Part print with two shaded views. Sizes in mm from the minimum x, y, z corner. A direction names the side the tool comes from. Give positions to 0.01 mm unless a question says otherwise; leave off trailing zeros. Loops run counter-clockwise (first coordinate to the right, second up) from the corner with the lowest first, then second, coordinate; pieces in that order, holes last. Notation, with made-up numbers: (63.5, -27) -> (111.5, -27) arc R20 ccw to (111.5, -10) -> close; hole circle Ø7 at (-33, -40). An arc over 180 degrees is marked (long way). One line per question, with ' | ' between items.
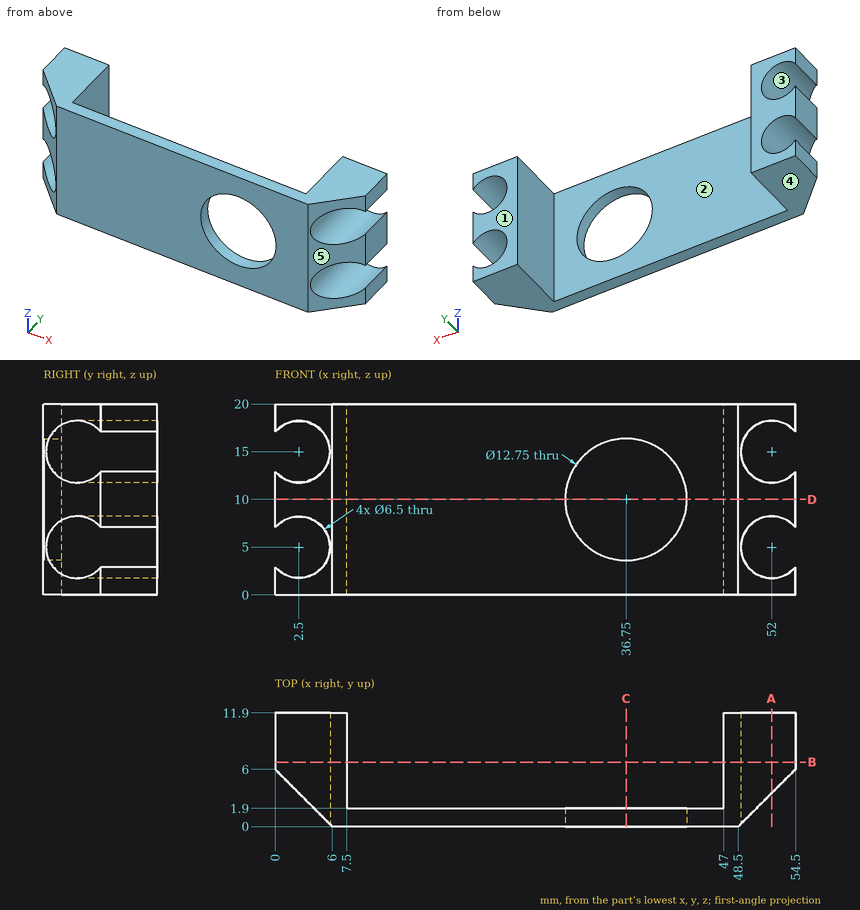
1) Pull direction Z, two halves, no side cores. Call the marked faces 3, 4 and 5: pulls with the +Z half, pulls with the -Z half, needs draft (parallel to the pull), parting line crosses it, or undercut.
Found:
face 3: undercut | face 4: pulls with the -Z half | face 5: needs draft
2) Tool access for the marked faces 1 and 2: list every direction of +Z, -Z, +X, -X, +Y, -Y with a clear straight run to the whole face (end or side of a thin tool).
Found:
face 1: +Z, -Z, +X, -X, +Y | face 2: +Z, -Z, +Y
3) Drill centre lines: line 1 (Z direction, x = 52, y = 6.75); line 2 (X direction, y = 4.5, z = 15); line 3 (X direction, y = 10.75, z = 7.5). Where is each one in solid material? Low to high.
Found:
line 1: 0 to 1.75, 8.25 to 11.75, 18.25 to 20 | line 2: 5.75 to 7.5, 47 to 48.75 | line 3: 0 to 0.42, 4.58 to 7.5, 47 to 49.92, 54.08 to 54.5
4) Pin check, flat tips, straight feed: P1, Ø6, axis at x = 28, z = 4.5, coming from the +Y side; P2, Ø3, axis at y = 8.5, z = 15, coming from the -X side; P3, Ø4, axis at y = 7, z = 5, coming from the +X side. Stop position of each tip, or through.
Found:
P1: y = 1.9 | P2: x = 5.38 | P3: x = 49.44
5) Saw through at D-D (z = 10). Give the cut face in (x, y) (3 decimals), and give its area (3 significant figures).
Found:
outline: (0, 6) -> (6, 0) -> (30.375, 0) -> (30.375, 1.9) -> (7.5, 1.9) -> (7.5, 11.9) -> (0, 11.9) -> close; (43.125, 0) -> (48.5, 0) -> (54.5, 6) -> (54.5, 11.9) -> (47, 11.9) -> (47, 1.9) -> (43.125, 1.9) -> close | area: 193 mm2
6) Saw through at C-C (x = 36.75). Give the cut face in (y, z) (3 decimals).
Found:
outline: (0, 0) -> (1.9, 0) -> (1.9, 3.625) -> (0, 3.625) -> close; (0, 16.375) -> (1.9, 16.375) -> (1.9, 20) -> (0, 20) -> close
7) Saw through at A-A (x = 52). Give the cut face in (y, z).
Found:
outline: (3.5, 0) -> (11.9, 0) -> (11.9, 1.75) -> (3.5, 1.75) -> close; (3.5, 8.25) -> (11.9, 8.25) -> (11.9, 11.75) -> (3.5, 11.75) -> close; (3.5, 18.25) -> (11.9, 18.25) -> (11.9, 20) -> (3.5, 20) -> close
8) Saw through at B-B (y = 6.75). Give the cut face in (x, z), and give its area (3 significant figures).
Found:
outline: (0, 0) -> (7.5, 0) -> (7.5, 20) -> (0, 20) -> (0, 17.08) arc R3.25 cw (long way) to (0, 12.92) -> (0, 7.08) arc R3.25 cw (long way) to (0, 2.92) -> close; (47, 0) -> (54.5, 0) -> (54.5, 2.92) arc R3.25 cw (long way) to (54.5, 7.08) -> (54.5, 12.92) arc R3.25 cw (long way) to (54.5, 17.08) -> (54.5, 20) -> (47, 20) -> close | area: 176 mm2
